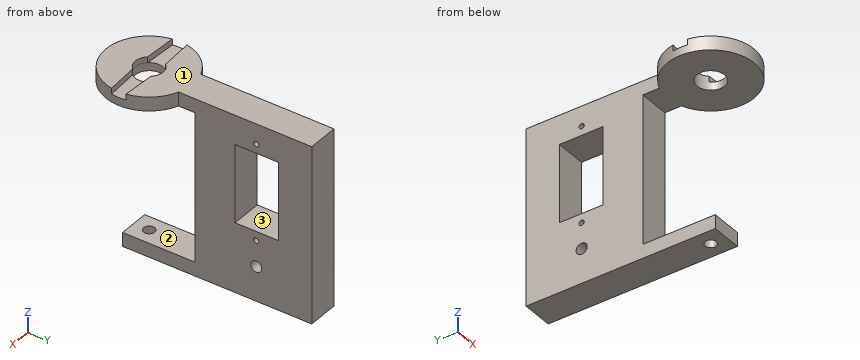
from build123d import *

# Parameters (mm, degrees)
SKETCH1_R           = 12.5
SKETCH1_R_2         = 4
BOSS_EXTRUDE1_DEPTH = 4
CUT_EXTRUDE1_DEPTH  = 1.7
SKETCH3_W           = 8.958376624
SKETCH3_H           = 30
BOSS_EXTRUDE2_DEPTH = 4
SKETCH4_W           = 8.958376624
SKETCH4_H           = 24.069748571
BOSS_EXTRUDE3_DEPTH = 47
SKETCH5_W           = 8.958376624
SKETCH5_H           = 45
SKETCH5_R           = 1.6
BOSS_EXTRUDE4_DEPTH = 4
SKETCH6_W           = 22.5
SKETCH6_H           = 12.5
CUT_EXTRUDE2_DEPTH  = 68.301878397
SKETCH7_R           = 1.6
CUT_EXTRUDE3_DEPTH  = 68.301878397
SKETCH8_R           = 0.75
CUT_EXTRUDE4_DEPTH  = 68.301878397
SKETCH9_W           = 51
SKETCH9_H           = 9.652107549
BOSS_EXTRUDE5_DEPTH = 8.95837662


with BuildPart() as part:
    # Sketch1 → Boss-Extrude1 (new body)
    with BuildSketch(Plane.XY):
        Circle(SKETCH1_R)
        Circle(SKETCH1_R_2, mode=Mode.SUBTRACT)
    extrude(amount=-BOSS_EXTRUDE1_DEPTH)

    # Sketch2 → Cut-Extrude1 (cut)
    with BuildSketch(Plane.XY):
        with BuildLine():
            Line((14.05, 2), (3.035592941, 2.604836943))
            ThreePointArc((3.035592941, 2.604836943), (0, 4), (-3.035592941, 2.604836943))
            Line((-3.035592941, 2.604836943), (-14.05, 2))
            ThreePointArc((-14.05, 2), (-16.05, 0), (-14.05, -2))
            Line((-14.05, -2), (-3.035592941, -2.604836943))
            ThreePointArc((-3.035592941, -2.604836943), (0, -4), (3.035592941, -2.604836943))
            Line((3.035592941, -2.604836943), (14.05, -2))
            ThreePointArc((14.05, -2), (16.05, 0), (14.05, 2))
        make_face()
    extrude(amount=-CUT_EXTRUDE1_DEPTH, mode=Mode.SUBTRACT)

    # Sketch3 → Boss-Extrude2 (add)
    with BuildSketch(Plane.XY):
        with Locations((0, 25.5)):
            Rectangle(SKETCH3_W, SKETCH3_H)
    extrude(amount=-BOSS_EXTRUDE2_DEPTH)

    # Sketch4 → Boss-Extrude3 (add)
    with BuildSketch(Plane(origin=(0, 0, -4), x_dir=(-1, 0, 0), z_dir=(0, 0, -1))):
        with Locations((0, 28.465125715)):
            Rectangle(SKETCH4_W, SKETCH4_H)
    extrude(amount=BOSS_EXTRUDE3_DEPTH)

    # Sketch5 → Boss-Extrude4 (add)
    with BuildSketch(Plane(origin=(0, 0, -51), x_dir=(-1, 0, 0), z_dir=(0, 0, -1))):
        with Locations((0, 18)):
            Rectangle(SKETCH5_W, SKETCH5_H)
        Circle(SKETCH5_R, mode=Mode.SUBTRACT)
    extrude(amount=-BOSS_EXTRUDE4_DEPTH)

    # Sketch6 → Cut-Extrude2 (cut, through all)
    with BuildSketch(Plane(origin=(4.479188312, 0, 0), x_dir=(0, 0, -1), z_dir=(1, 0, 0))):
        with Locations((19.677937554, 34.25)):
            Rectangle(SKETCH6_W, SKETCH6_H)
    extrude(amount=-CUT_EXTRUDE2_DEPTH, mode=Mode.SUBTRACT)

    # Sketch7 → Cut-Extrude3 (cut, through all)
    with BuildSketch(Plane(origin=(4.479188312, 0, 0), x_dir=(0, 0, -1), z_dir=(1, 0, 0))):
        with Locations(Location((41.027937554, 34.1, 0), (0, 0, 90))):
            Circle(SKETCH7_R)
    extrude(amount=-CUT_EXTRUDE3_DEPTH, mode=Mode.SUBTRACT)

    # Sketch8 → Cut-Extrude4 (cut, through all)
    with BuildSketch(Plane.ZY.offset(4.479188312)):
        with Locations(Location((-33.577937554, 34.1, 0), (0, 0, 270))):
            Circle(SKETCH8_R)
        with Locations(Location((-5.777937554, 34.1, 0), (0, 0, 270))):
            Circle(SKETCH8_R)
    extrude(amount=-CUT_EXTRUDE4_DEPTH, mode=Mode.SUBTRACT)

    # Sketch9 → Boss-Extrude5 (add)
    with BuildSketch(Plane(origin=(4.479188312, 0, 0), x_dir=(0, 0, -1), z_dir=(1, 0, 0))):
        with Locations((25.5, 45.326053774)):
            Rectangle(SKETCH9_W, SKETCH9_H)
    extrude(amount=-BOSS_EXTRUDE5_DEPTH)


solid = part.part
Build history of the part. All positions in model axes, mm. Face numbers are marked on the shaded views. A direction names the side the tool comes from. Coordinates: 2 decimals unless noted, no trailing zeros. Write each loop counter-clockwise with the first axis right and the second up, starting at its lowest first coordinate (ties: lowest second). Pieces come first, ordered by that corner, then holes. Notation, with made-up numbers: (50.25, -39) -> (94.25, -39) arc R14 cw to (94.25, -19) -> close; hole circle Ø5 at (58.5, -12). An arc over 180 degrees is marked (long way). Use CSV: the item, a comma, the result in double quotes. Start each with the question number.
Q1. Drill centre lines: probe 1 along Z at (x, y) = (-1.25, 34.1); probe 2 along Z at (x, y) = (-3, 3.5); probe 3 along Y at (x, z) = (3.25, -19). Where is each one in solid material? Low to high.
Q2. Cut at A-A, the plane z = -13.5. List the corners of the cut face in (x, y), then the cut area to 3 significant figures.
Q3. Cut at B-B, the plane y = 37.5. List the corners of the cut face in (x, z), then the cut area to 3 significant figures.
Q4. Cut at C-C, the plane x = 0. List the corners of the cut face in (y, z).
Q5. Flat gauge pins, fed straight in: pin 1 Ø7 at (x, z) = (0.5, -19) entering from -Y; pin 2 Ø0.9 at (y, z) = (34.1, -5.78) entering from -X; pin 3 Ø1.6 at (x, y) = (9, 0) entering from +Z; pin 4 Ø5 at (y, z) = (22.5, -26) entering from -X. Where does each tip first touch, or does it go through?
Q6. Cut at D-D, the plane y = 0. List the corners of the cut face in (x, z), then the cut area to 3 significant figures.
Q7. 3-axis set-ups, long thin cutter, end or side, ignore diameter. For the marked faces 1, 2 and 3: which of +Z, -Z, +X, -X, +Y, -Y reach the whole face in a straight line?
Checked values:
1,probe 1,"z = -51 to -42.63, -39.43 to -34.33, -32.83 to -30.93, -8.43 to -6.53, -5.03 to 0"
1,probe 2,"z = -51 to -47, -4 to 0"
1,probe 3,"y = 16.43 to 28, 40.5 to 50.15"
2,outline,"(-4.48, 16.43) -> (4.48, 16.43) -> (4.48, 28) -> (-4.48, 28) -> close; (-4.48, 40.5) -> (4.48, 40.5) -> (4.48, 50.15) -> (-4.48, 50.15) -> close"
2,area,"190 mm²"
3,outline,"(-4.48, -51) -> (4.48, -51) -> (4.48, -30.93) -> (-4.48, -30.93) -> close; (-4.48, -8.43) -> (4.48, -8.43) -> (4.48, 0) -> (-4.48, 0) -> close"
3,area,"255 mm²"
4,outline,"(-12.5, -4) -> (-4, -4) -> (-4, 0) -> (-12.5, 0) -> close; (-4.5, -51) -> (-1.6, -51) -> (-1.6, -47) -> (-4.5, -47) -> close; (1.6, -51) -> (50.15, -51) -> (50.15, 0) -> (4, 0) -> (4, -4) -> (16.43, -4) -> (16.43, -47) -> (1.6, -47) -> close; hole (28, -30.93) -> (40.5, -30.93) -> (40.5, -8.43) -> (28, -8.43) -> close; hole circle Ø3.2 at (34.1, -41.03); hole circle Ø1.5 at (34.1, -33.58); hole circle Ø1.5 at (34.1, -5.78)"
5,pin 1,"stops at y = 16.43"
5,pin 2,"passes through"
5,pin 3,"stops at z = -1.7"
5,pin 4,"stops at x = -4.48"
6,outline,"(-12.5, -4) -> (-4, -4) -> (-4, -1.7) -> (-12.5, -1.7) -> close; (-4.48, -51) -> (-1.6, -51) -> (-1.6, -47) -> (-4.48, -47) -> close; (1.6, -51) -> (4.48, -51) -> (4.48, -47) -> (1.6, -47) -> close; (4, -4) -> (12.5, -4) -> (12.5, -1.7) -> (4, -1.7) -> close"
6,area,"62.1 mm²"
7,face 1,"+Z, +X, -X, +Y, -Y"
7,face 2,"+X, -X, -Y"
7,face 3,"+X, -X"
